CAD build for the part. Positions are in the model's coordinates, mm. Face numbers are marked on the shaded views. A direction names the side the tool comes from. Round coordinates to 2 decimals unless told otherwise and drop trailing zeros. Put each result on its own line as item: value. Start each with the question number.
Item 1: Drill centre lines: line 1 (Z direction, x = -14, y = 4.25); line 2 (X direction, y = 7.25, z = 17.5); line 3 (Z direction, x = -27, y = 14.25). Where is each one in solid material? Low to high. Write a range as from..to.
Item 2: Pin check, flat tips, straight feed: pin 1 Ø1 at (x, z) = (-47.5, 1.5) entering from -Y; pin 2 Ø3 at (x, z) = (37.5, -35) entering from -Y; pin 3 Ø8 at (x, z) = (-48.01, -44.53) entering from -Y (3 decimals); pin 4 Ø4 at (x, z) = (50, -11.5) entering from +Y (3 decimals). Stop position of each tip, or through.
Item 3: Mould opens along Z. For the marked faces 3, 4 and 5 say: released by +Z, released by -Z, zero draft, split by the parting line, or undercut.
Item 4: Cut at A-A (z = 0). Count the separate pieces of the cut face and the enclosed holes in it, and give its area (3 significant figures).
Item 5: 3-axis set-ups, long thin cutter, end or side, ignore diameter. For the marked faces 1 and 2: which of +Z, -Z, +X, -X, +Y, -Y reach the whole face in a straight line?
```python
from build123d import *

# Parameters (mm, degrees)
SKETCH2_W                      = 134.112
SKETCH2_H                      = 127.1524
SKETCH2_W_2                    = 83.312
SKETCH2_H_2                    = 76.3524
SKETCH2_W_3                    = 21.7424
SKETCH2_H_3                    = 15.9766
BOSS_EXTRUDE1_DEPTH            = 15.875
BOSS_EXTRUDE2_DEPTH            = 9.525
CUT_EXTRUDE2_DEPTH             = 3.175
M2_5X0_45_TAPPED_HOLE1_D       = 2.05
M2_5X0_45_TAPPED_HOLE1_DEPTH   = 6.35
M2_5X0_45_TAPPED_HOLE1_TIP     = 0.615882135
F_10_CLEARANCE_HOLE1_D         = 5.1054
CUT_EXTRUDE3_DEPTH             = 6.35
CUT_EXTRUDE4_DEPTH             = 1.6
SKETCH12_W                     = 70.612
SKETCH12_H                     = 63.6524
CUT_EXTRUDE5_DEPTH             = 12.1
FILLET1_R                      = 3.81
SKETCH13_W                     = 134.112
SKETCH13_H                     = 127.1524
CUT_EXTRUDE6_DEPTH             = 1.5875
FILLET2_R                      = 1.5875
SKETCH14_W                     = 15.3924
SKETCH14_H                     = 22.86
CUT_EXTRUDE7_DEPTH             = 4.75
FILLET3_R                      = 3.175
SKETCH15_W                     = 134.112
SKETCH15_H                     = 127.1524
BOSS_EXTRUDE3_DEPTH            = 3.175
F_6_32_TAPPED_HOLE1_AT_2_COUNT = 2
F_6_32_TAPPED_HOLE1_AT_2_PITCH = 108.1024
F_6_32_TAPPED_HOLE1_AT_3_COUNT = 2
F_6_32_TAPPED_HOLE1_AT_3_PITCH = 85.702359025
F_6_32_TAPPED_HOLE1_AT_4_COUNT = 2
F_6_32_TAPPED_HOLE1_AT_4_PITCH = 43.049882955
SKETCH19_R                     = 2.7813
CUT_EXTRUDE8_DEPTH             = 3.175
F_4_40_TAPPED_HOLE1_D          = 2.2606
F_4_40_TAPPED_HOLE1_DEPTH      = 7.62
F_4_40_TAPPED_HOLE1_TIP        = 0.679152758


with BuildPart() as part:
    # Sketch2 → Boss-Extrude1 (new body)
    with BuildSketch(Plane(origin=(0, 0, 0), x_dir=(1, 0, 0), z_dir=(0, 1, 0))):
        Rectangle(SKETCH2_W, SKETCH2_H)
        Rectangle(SKETCH2_W_2, SKETCH2_H_2, mode=Mode.SUBTRACT)
        with Locations((-30.7848, 30.1879)):
            Rectangle(SKETCH2_W_3, SKETCH2_H_3)
    extrude(amount=BOSS_EXTRUDE1_DEPTH)

    # Sketch4 → Boss-Extrude2 (add)
    with BuildSketch(Plane(origin=(0, 0, 0), x_dir=(1, 0, 0), z_dir=(0, 1, 0))):
        Polygon((41.656, -38.1762), (41.656, 38.1762), (-19.9136, 38.1762), (-19.9136, 22.1996), (-41.656, 22.1996), (-41.656, -38.1762), align=None)
        Polygon((35.306, 31.8262), (-13.5636, 31.8262), (-13.5636, 15.8496), (-35.306, 15.8496), (-35.306, -31.8262), (35.306, -31.8262), align=None, mode=Mode.SUBTRACT)
    extrude(amount=BOSS_EXTRUDE2_DEPTH)

    # Sketch5 → Cut-Extrude2 (cut)
    with BuildSketch(Plane.XZ):
        with BuildLine():
            Line((46.736, -50.8762), (-46.736, -50.8762))
            ThreePointArc((-46.736, -50.8762), (-52.124153673, -48.644353673), (-54.356, -43.2562))
            Line((-54.356, -43.2562), (-54.356, 43.2562))
            ThreePointArc((-54.356, 43.2562), (-52.124153673, 48.644353673), (-46.736, 50.8762))
            Line((-46.736, 50.8762), (46.736, 50.8762))
            ThreePointArc((46.736, 50.8762), (52.124153673, 48.644353673), (54.356, 43.2562))
            Line((54.356, 43.2562), (54.356, -43.2562))
            ThreePointArc((54.356, -43.2562), (52.124153673, -48.644353673), (46.736, -50.8762))
        make_face()
    extrude(amount=-CUT_EXTRUDE2_DEPTH, mode=Mode.SUBTRACT)

    # M2.5x0.45 Tapped Hole1
    with Locations(Plane(origin=(0, 3.175, 0), x_dir=(-1, 0, 0), z_dir=(0, -1, 0))):
        with Locations((38.481, -35.0012), (-38.481, -35.0012), (38.481, 19.0246), (16.7386, 35.0012), (-38.481, 35.0012)):
            Hole(M2_5X0_45_TAPPED_HOLE1_D / 2, depth=M2_5X0_45_TAPPED_HOLE1_DEPTH)
            with Locations((0, 0, -(M2_5X0_45_TAPPED_HOLE1_DEPTH + M2_5X0_45_TAPPED_HOLE1_TIP / 2))):  # 118° drill point
                Cone(0, M2_5X0_45_TAPPED_HOLE1_D / 2, M2_5X0_45_TAPPED_HOLE1_TIP, mode=Mode.SUBTRACT)

    # #10 Clearance Hole1 (through all)
    with Locations(Plane(origin=(0, 3.175, 0), x_dir=(-1, 0, 0), z_dir=(0, -1, 0))):
        with Locations((48.006, -44.5262), (0, -44.5262), (-48.006, -44.5262), (-48.006, 0), (-48.006, 44.5262), (0, 44.5262), (48.006, 44.5262), (48.006, 0)):
            Hole(F_10_CLEARANCE_HOLE1_D / 2)

    # Sketch10 → Cut-Extrude3 (cut)
    with BuildSketch(Plane(origin=(0, 15.875, 0), x_dir=(1, 0, 0), z_dir=(0, 1, 0))):
        with BuildLine():
            Line((54.356, -43.2562), (54.356, 43.2562))
            ThreePointArc((54.356, 43.2562), (52.124153673, 48.644353673), (46.736, 50.8762))
            Line((46.736, 50.8762), (-46.736, 50.8762))
            ThreePointArc((-46.736, 50.8762), (-52.124153673, 48.644353673), (-54.356, 43.2562))
            Line((-54.356, 43.2562), (-54.356, -43.2562))
            ThreePointArc((-54.356, -43.2562), (-52.124153673, -48.644353673), (-46.736, -50.8762))
            Line((-46.736, -50.8762), (46.736, -50.8762))
            ThreePointArc((46.736, -50.8762), (52.124153673, -48.644353673), (54.356, -43.2562))
        make_face()
    extrude(amount=-CUT_EXTRUDE3_DEPTH, mode=Mode.SUBTRACT)

    # Sketch11 → Cut-Extrude4 (cut)
    with BuildSketch(Plane.XZ.offset(-3.175)):
        with BuildLine():
            Line((40.513, 40.2082), (-40.513, 40.2082))
            ThreePointArc((-40.513, 40.2082), (-42.75806403, 39.27826403), (-43.688, 37.0332))
            Line((-43.688, 37.0332), (-43.688, -37.0332))
            ThreePointArc((-43.688, -37.0332), (-42.75806403, -39.27826403), (-40.513, -40.2082))
            Line((-40.513, -40.2082), (40.513, -40.2082))
            ThreePointArc((40.513, -40.2082), (42.75806403, -39.27826403), (43.688, -37.0332))
            Line((43.688, -37.0332), (43.688, 37.0332))
            ThreePointArc((43.688, 37.0332), (42.75806403, 39.27826403), (40.513, 40.2082))
        make_face()
    extrude(amount=-CUT_EXTRUDE4_DEPTH, mode=Mode.SUBTRACT)

    # Sketch12 → Cut-Extrude5 (cut, through all)
    with BuildSketch(Plane.XZ.offset(-4.775)):
        Rectangle(SKETCH12_W, SKETCH12_H)
    extrude(amount=-CUT_EXTRUDE5_DEPTH, mode=Mode.SUBTRACT)

    # Fillet1
    fillet1_edges = [part.edges().sort_by_distance(p)[0] for p in [
        (-35.306, 7.15, -31.8262),
        (35.306, 7.15, -31.8262),
        (-35.306, 7.15, 31.8262),
        (35.306, 7.15, 31.8262),
    ]]
    fillet(fillet1_edges, radius=FILLET1_R)

    # Sketch13 → Cut-Extrude6 (cut)
    with BuildSketch(Plane.XZ):
        Rectangle(SKETCH13_W, SKETCH13_H)
        with BuildLine():
            Line((54.356, -43.2562), (54.356, 43.2562))
            ThreePointArc((54.356, 43.2562), (52.124153673, 48.644353673), (46.736, 50.8762))
            Line((46.736, 50.8762), (-46.736, 50.8762))
            ThreePointArc((-46.736, 50.8762), (-52.124153673, 48.644353673), (-54.356, 43.2562))
            Line((-54.356, 43.2562), (-54.356, -43.2562))
            ThreePointArc((-54.356, -43.2562), (-52.124153673, -48.644353673), (-46.736, -50.8762))
            Line((-46.736, -50.8762), (46.736, -50.8762))
            ThreePointArc((46.736, -50.8762), (52.124153673, -48.644353673), (54.356, -43.2562))
        make_face(mode=Mode.SUBTRACT)
    extrude(amount=-CUT_EXTRUDE6_DEPTH, mode=Mode.SUBTRACT)

    # Fillet2
    fillet2_edges = [part.edges().sort_by_distance(p)[0] for p in [
        (67.056, 1.5875, 0),
        (0, 1.5875, -63.5762),
        (-67.056, 1.5875, 0),
        (0, 1.5875, 63.5762),
    ]]
    fillet(fillet2_edges, radius=FILLET2_R)

    # Sketch14 → Cut-Extrude7 (cut)
    with BuildSketch(Plane(origin=(0, 9.525, 0), x_dir=(1, 0, 0), z_dir=(0, 1, 0))):
        with Locations((-27.6098, 39.4462)):
            Rectangle(SKETCH14_W, SKETCH14_H)
    extrude(amount=-CUT_EXTRUDE7_DEPTH, mode=Mode.SUBTRACT)

    # Fillet3
    fillet3_edges = [part.edges().sort_by_distance(p)[0] for p in [
        (-19.9136, 7.15, -31.8262),
        (-19.9136, 7.15, -50.8762),
        (-35.306, 7.15, -50.8762),
    ]]
    fillet(fillet3_edges, radius=FILLET3_R)

    # Sketch15 → Boss-Extrude3 (add)
    with BuildSketch(Plane(origin=(0, 15.875, 0), x_dir=(1, 0, 0), z_dir=(0, 1, 0))):
        Rectangle(SKETCH15_W, SKETCH15_H)
        with BuildLine():
            ThreePointArc((46.736, -57.2262), (56.614281733, -53.134481733), (60.706, -43.2562))
            Line((60.706, -43.2562), (60.706, 43.2562))
            ThreePointArc((60.706, 43.2562), (56.614281733, 53.134481733), (46.736, 57.2262))
            Line((46.736, 57.2262), (-46.736, 57.2262))
            ThreePointArc((-46.736, 57.2262), (-56.614281733, 53.134481733), (-60.706, 43.2562))
            Line((-60.706, 43.2562), (-60.706, -43.2562))
            ThreePointArc((-60.706, -43.2562), (-56.614281733, -53.134481733), (-46.736, -57.2262))
            Line((-46.736, -57.2262), (46.736, -57.2262))
        make_face(mode=Mode.SUBTRACT)
    extrude(amount=BOSS_EXTRUDE3_DEPTH)

    # Sketch18 → #6-32 Tapped Hole1 (revolve, cut)
    with BuildSketch(Plane(origin=(-25.4, 15.875, 54.0512), x_dir=(0, 0, 1), z_dir=(1, 0, 0))):
        Polygon((0, 0), (0, 10.33769403), (1.35255, 9.525), (1.35255, 0), align=None)
    f_6_32_tapped_hole1 = revolve(axis=Axis((-25.4, 22.225, 54.0512), (0, -1, 0)), mode=Mode.SUBTRACT)

    # #6-32 Tapped Hole1 at 2: #6-32 Tapped Hole1 ×2
    with Locations(*[(0, 0, -i * F_6_32_TAPPED_HOLE1_AT_2_PITCH) for i in range(1, F_6_32_TAPPED_HOLE1_AT_2_COUNT)]):
        add(f_6_32_tapped_hole1, mode=Mode.SUBTRACT)

    # #6-32 Tapped Hole1 at 3: #6-32 Tapped Hole1 ×2
    with Locations(*[Vector(-0.374913834, 0, -0.927059662) * (i * F_6_32_TAPPED_HOLE1_AT_3_PITCH) for i in range(1, F_6_32_TAPPED_HOLE1_AT_3_COUNT)]):
        add(f_6_32_tapped_hole1, mode=Mode.SUBTRACT)

    # #6-32 Tapped Hole1 at 4: #6-32 Tapped Hole1 ×2
    with Locations(*[Vector(-0.746366721, 0, -0.665534911) * (i * F_6_32_TAPPED_HOLE1_AT_4_PITCH) for i in range(1, F_6_32_TAPPED_HOLE1_AT_4_COUNT)]):
        add(f_6_32_tapped_hole1, mode=Mode.SUBTRACT)

    # Mirror1: #6-32 Tapped Hole1 across plane
    add(f_6_32_tapped_hole1.mirror(Plane(origin=(0, 0, 0), x_dir=(0, 0, 1), z_dir=(1, 0, 0))), mode=Mode.SUBTRACT)

    # Mirror1 copy 1 sketch → Mirror1 copy 1 (revolve, cut)
    with BuildSketch(Plane(origin=(25.4, 15.875, -54.0512), x_dir=(0, 0, 1), z_dir=(-1, 0, 0))):
        Polygon((0, 0), (0, -10.33769403), (1.35255, -9.525), (1.35255, 0), align=None)
    revolve(axis=Axis((25.4, 22.225, -54.0512), (0, 1, 0)), mode=Mode.SUBTRACT)

    # Mirror1 copy 2 sketch → Mirror1 copy 2 (revolve, cut)
    with BuildSketch(Plane(origin=(57.531, 15.875, -25.4), x_dir=(0, 0, 1), z_dir=(-1, 0, 0))):
        Polygon((0, 0), (0, -10.33769403), (1.35255, -9.525), (1.35255, 0), align=None)
    revolve(axis=Axis((57.531, 22.225, -25.4), (0, 1, 0)), mode=Mode.SUBTRACT)

    # Mirror1 copy 3 sketch → Mirror1 copy 3 (revolve, cut)
    with BuildSketch(Plane(origin=(57.531, 15.875, 25.4), x_dir=(0, 0, 1), z_dir=(-1, 0, 0))):
        Polygon((0, 0), (0, -10.33769403), (1.35255, -9.525), (1.35255, 0), align=None)
    revolve(axis=Axis((57.531, 22.225, 25.4), (0, 1, 0)), mode=Mode.SUBTRACT)

    # Sketch19 → Cut-Extrude8 (cut)
    with BuildSketch(Plane.XZ.offset(-4.775)):
        with Locations((38.481, 35.0012)):
            Circle(SKETCH19_R)
        with Locations((38.481, -35.0012)):
            Circle(SKETCH19_R)
        with Locations((-38.481, 35.0012)):
            Circle(SKETCH19_R)
        with Locations((-38.481, -19.0246)):
            Circle(SKETCH19_R)
        with Locations((-16.7386, -35.0012)):
            Circle(SKETCH19_R)
    extrude(amount=-CUT_EXTRUDE8_DEPTH, mode=Mode.SUBTRACT)

    # #4-40 Tapped Hole1
    with Locations(Plane(origin=(0, 9.525, 0), x_dir=(1, 0, 0), z_dir=(0, 1, 0))):
        with Locations((-38.481, 19.0246), (-16.7386, 35.0012), (38.481, 35.0012), (38.481, -35.0012), (-38.481, -35.0012)):
            Hole(F_4_40_TAPPED_HOLE1_D / 2, depth=F_4_40_TAPPED_HOLE1_DEPTH)
            with Locations((0, 0, -(F_4_40_TAPPED_HOLE1_DEPTH + F_4_40_TAPPED_HOLE1_TIP / 2))):  # 118° drill point
                Cone(0, F_4_40_TAPPED_HOLE1_D / 2, F_4_40_TAPPED_HOLE1_TIP, mode=Mode.SUBTRACT)


solid = part.part
```
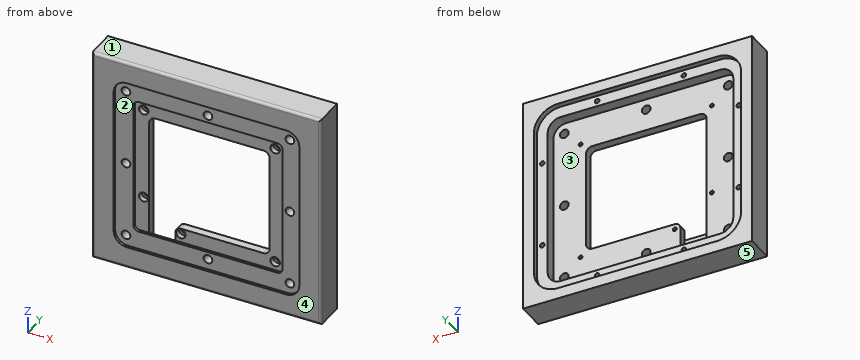
Output values:
1. line 1: -63.58..-40.21, 40.21..63.58
1. line 2: -67.06..-35.31, 35.31..67.06
1. line 3: -63.58..-50.88, 50.88..63.58
2. pin 1: through
2. pin 2: y = 7.95
2. pin 3: y = 3.175
2. pin 4: y = 9.525
3. face 3: undercut
3. face 4: zero draft
3. face 5: released by -Z
4. separate pieces: 4
4. enclosed holes: 0
4. area: 552 mm2
5. face 1: +Z, +X, -X, +Y, -Y
5. face 2: -Y
